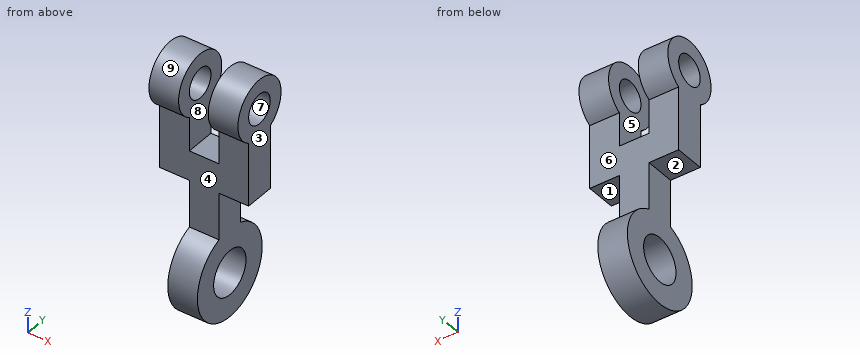
from build123d import *

# Parameters (mm, degrees)
SKETCH1_R           = 19.05
SKETCH1_R_2         = 9.525
BOSS_EXTRUDE1_DEPTH = 6.35
SKETCH1_3_W         = 12.7
SKETCH1_3_H         = 12.7
BOSS_EXTRUDE2_DEPTH = 19.05
BOSS_EXTRUDE3_START = 6.35
SKETCH1_4_R         = 12.7
SKETCH1_4_R_2       = 6.35
BOSS_EXTRUDE3_DEPTH = 12.7


with BuildPart() as part:
    # Sketch1 → Boss-Extrude1 (new, symmetric)
    with BuildSketch(Plane(origin=(0, 0, 0), x_dir=(0, 0, -1), z_dir=(1, 0, 0))):
        with Locations((76.2, 0)):
            Circle(SKETCH1_R)
        with Locations((76.2, 0)):
            Circle(SKETCH1_R_2, mode=Mode.SUBTRACT)
        with BuildLine():
            Line((38.1, 6.35), (38.1, -6.35))
            Line((38.1, -6.35), (58.239487758, -6.35))
            ThreePointArc((58.239487758, -6.35), (57.15, 0), (58.239487758, 6.35))
            Line((58.239487758, 6.35), (38.1, 6.35))
        make_face()
    extrude(amount=BOSS_EXTRUDE1_DEPTH, both=True)

    # Sketch1_3 → Boss-Extrude2 (add, symmetric)
    with BuildSketch(Plane(origin=(0, 0, 0), x_dir=(0, 0, -1), z_dir=(1, 0, 0))):
        with Locations((31.75, 0)):
            Rectangle(SKETCH1_3_W, SKETCH1_3_H)
    extrude(amount=BOSS_EXTRUDE2_DEPTH, both=True)


with BuildPart() as body_2:
    # Sketch1_4 → Boss-Extrude3 (new body)
    with BuildSketch(Plane(origin=(0, 0, 0), x_dir=(0, 0, -1), z_dir=(1, 0, 0)).offset(BOSS_EXTRUDE3_START)):
        with BuildLine():
            ThreePointArc((12.7, 0), (12.267257994, -3.287001873), (10.998522628, -6.35))
            Line((10.998522628, -6.35), (25.4, -6.35))
            Line((25.4, -6.35), (25.4, 6.35))
            Line((25.4, 6.35), (10.998522628, 6.35))
            ThreePointArc((10.998522628, 6.35), (12.267257994, 3.287001873), (12.7, 0))
        make_face()
        Circle(SKETCH1_4_R)
        Circle(SKETCH1_4_R_2, mode=Mode.SUBTRACT)
    boss_extrude3 = extrude(amount=BOSS_EXTRUDE3_DEPTH)


with BuildPart() as part_1:
    add(part.part)

    # Mirror2: Boss-Extrude3 across plane
    add(boss_extrude3.mirror(Plane(origin=(0, 0, 0), x_dir=(0, 0, 1), z_dir=(1, 0, 0))))


with BuildPart() as body_2_1:
    add(body_2.part)

    # Combine1: union part
    add(part_1.part)


solid = body_2_1.part
Here's how the part is built. I have some questions about the finished solid (model axes, mm). Face numbers are marked on the shaded views. A direction names the side the tool comes from. Round coordinates to 2 decimals unless told otherwise and drop trailing zeros. Loops run counter-clockwise (first coordinate to the right, second up) from the corner with the lowest first, then second, coordinate; pieces in that order, holes last.
1. If we section it at B-B on y = 0: Write out the boundary of the cut face in (x, z) (3 decimals), plus the area to 3 significant figures.
Answer list:
outline: (-19.05, -38.1) - (-6.35, -38.1) - (-6.35, -66.675) - (6.35, -66.675) - (6.35, -38.1) - (19.05, -38.1) - (19.05, -6.35) - (6.35, -6.35) - (6.35, -25.4) - (-6.35, -25.4) - (-6.35, -6.35) - (-19.05, -6.35) - close; (-19.05, 6.35) - (-6.35, 6.35) - (-6.35, 12.7) - (-19.05, 12.7) - close; (-6.35, -95.25) - (6.35, -95.25) - (6.35, -85.725) - (-6.35, -85.725) - close; (6.35, 6.35) - (19.05, 6.35) - (19.05, 12.7) - (6.35, 12.7) - close
area: 1,610 mm2
2. Which directions (+Z, -Z, +X, -X, +Y, -Y) give clear straight access to the entire face, cutting with the end or side of a thin tool? Please do the marked faces 1, 2, 3, 4 and 5.
Answer list:
face 1: -Z, +X, +Y, -Y
face 2: -Z, -X, +Y, -Y
face 3: +Z, -Z, +X, +Y, -Y
face 4: +X, -X, -Y
face 5: +Z, +Y, -Y
3. For P1, Ø12, axis at y = -13, z = -84.5, coming from the +X side; P2, Ø11.5, axis at y = 4.5, z = -74, coming from the -X side; P3, Ø4, axis at x = 15, y = -1, coming from the -Z side, each with a flat end and sliding along its axis, tell me the tip position at first contact or that it passes through.
Answer list:
P1: stops at x = 6.35
P2: stops at x = -6.35
P3: stops at z = -38.1
4. If we section it at C-C on x = -3.5: Write out the boundary of the cut face in (y, z) (3 decimals), plus the area to 3 significant figures.
Answer list:
outline: (-6.35, -58.239) arc R19.05 ccw (long way) to (6.35, -58.239) - (6.35, -25.4) - (-6.35, -25.4) - close; hole circle Ø19.05 at (0, -76.2)
area: 1,260 mm2
5. If we section it at A-A on z = -76.2: Write out the boundary of the cut face in (x, y) (3 decimals).
Answer list:
outline: (-6.35, -19.05) - (6.35, -19.05) - (6.35, -9.525) - (-6.35, -9.525) - close; (-6.35, 9.525) - (6.35, 9.525) - (6.35, 19.05) - (-6.35, 19.05) - close
6. If we section it at D-D on z = 0: Write out the boundary of the cut face in (x, y).
Answer list:
outline: (-19.05, -12.7) - (-6.35, -12.7) - (-6.35, -6.35) - (-19.05, -6.35) - close; (-19.05, 6.35) - (-6.35, 6.35) - (-6.35, 12.7) - (-19.05, 12.7) - close; (6.35, -12.7) - (19.05, -12.7) - (19.05, -6.35) - (6.35, -6.35) - close; (6.35, 6.35) - (19.05, 6.35) - (19.05, 12.7) - (6.35, 12.7) - close
7. If I drill on line 1 along X through (y, z) = (4, -17.5); line 2 along Z through (x, y) = (-0.5, 0.5); line 3 along Y through (x, z) = (10.5, -15), over which ranges is the centre line in solid material (lowest first)?
Answer list:
line 1: x = -19.05 to -6.35, 6.35 to 19.05
line 2: z = -95.24 to -85.71, -66.69 to -25.4
line 3: y = -6.35 to 6.35
8. We'd pull the mould along Y, two halves only. Please class the marked faces 6, 7, 8 and 9: +Y half, -Y half, draft (parallel to the pull), parting line (faces both ways), or undercut.
Answer list:
face 6: +Y half
face 7: undercut
face 8: draft
face 9: parting line
